```python
from build123d import *

# Parameters (mm, degrees)
F0_W      = 152.4
F0_H      = 91.581002
F1_DEPTH  = 50.8
F2_R      = 19.05
F3_DEPTH  = 152.4
F2_R_2    = 22.225
F4_DEPTH  = 6.35
F5_R      = 22.225
F5_R_2    = 19.05
F6_DEPTH  = 6.35
F7_R      = 19.05
F8_DEPTH  = 82.55
F10_R     = 6.35
F11_DEPTH = 152.4
F12_R     = 6.35
F13_DEPTH = 38.1


with BuildPart() as f1:
    # F0 (on Right) → F1 (new body, symmetric)
    with BuildSketch(Plane.YZ):
        Rectangle(F0_W, F0_H)
    extrude(amount=F1_DEPTH, both=True)

    # F2 (on face) → F3 (cut, symmetric)
    with BuildSketch(Plane(origin=(0, 76.2, 0), x_dir=(-1, 0, 0), z_dir=(0, 1, 0))):
        Circle(F2_R)
    extrude(amount=F3_DEPTH, both=True, mode=Mode.SUBTRACT)

    # F2 (on face) → F4 (cut)
    with BuildSketch(Plane(origin=(0, 76.2, 0), x_dir=(-1, 0, 0), z_dir=(0, 1, 0))):
        Circle(F2_R_2)
        Circle(F2_R, mode=Mode.SUBTRACT)
    extrude(amount=-F4_DEPTH, mode=Mode.SUBTRACT)

    # F5 (on face) → F6 (cut)
    with BuildSketch(Plane.XZ.offset(76.2)):
        Circle(F5_R)
        Circle(F5_R_2, mode=Mode.SUBTRACT)
    extrude(amount=-F6_DEPTH, mode=Mode.SUBTRACT)

    # F7 (on Front) → F8 (join, symmetric)
    with BuildSketch(Plane.XZ):
        Circle(F7_R)
    extrude(amount=F8_DEPTH, both=True)

    # F10 (on face) → F11 (cut)
    with BuildSketch(Plane(origin=(-50.8, 0, 0), x_dir=(0, -1, 0), z_dir=(-1, 0, 0))):
        Circle(F10_R)
    extrude(amount=-F11_DEPTH, mode=Mode.SUBTRACT)

    # F12 (on Right) → F13 (join, symmetric)
    with BuildSketch(Plane.YZ):
        Circle(F12_R)
    extrude(amount=F13_DEPTH, both=True)


solid = f1.part
```
For this review, take the finished solid that the model builds, in its own axes (mm). A direction names the side the tool comes from. Round coordinates to 2 decimals unless told otherwise and drop trailing zeros. Write each loop counter-clockwise with the first axis right and the second up, starting at its lowest first coordinate (ties: lowest second). Pieces come first, ordered by that corner, then holes. Notation, with made-up numbers: (78.5, 21) - (120.5, 21) arc R8 cw to (120.5, 28) - close; hole circle Ø3 at (5.25, -27.5). An arc over 180 degrees is marked (long way). Answer as CSV lines item,"result". Start each with the question number.
(1) Machinability: for faces 4 (the flat face through (0, -82.55, 0)), 5 (the flat face through (-16.4, 69.85, 10)), 6 (the flat face through (38.1, 0, 0)), 7 (the cylindrical face through (-44.54, 1.38, -6.2)), 8 (the cylindrical face through (21.199, -73.069, 6.676)), which of the approach directions +Z, -Z, +X, -X, +Y, -Y give a long, thin tool a straight path to every point of the face, cutting with its end or side? Answer none if there is none.
(2) For line 1 (Y direction, x = 47, z = 0); line 2 (Z direction, x = -44, y = 0); line 3 (Z direction, x = 13.5, y = 71.5), list the stretches that pass through material, from the lowest coordinate up.
(3) For pin 1 (1.5 mm diameter, centred on x = -26.5, z = -19.5, fed in from -Y); pin 2 (10 mm diameter, centred on x = -37, z = -5, fed in from +Y); pin 3 (11.5 mm diameter, centred on y = 0, z = 0, fed in from -X); pin 4 (14 mm diameter, centred on y = -0.5, z = 2.5, fed in from +X), all flat-tipped, find the tip position at first contact; note any pin that passes through.
(4) Mouldability with a two-part tool opening along Z and no side actions: class faces 1 (the flat face through (23, 76.2, -1)), 2 (the flat face through (1, -1, 45.791)), 3 (the cylindrical face through (-21.199, 73.069, 6.676)) as +Z half, -Z half, draft (parallel to the pull), parting line (faces both ways), or undercut.
(5) Add section A-A, the plane y = 0. State the section outline as (x, z) points, plus the area to 3 significant figures.
(6) Add section D-D, the plane z = 32.5. State the section outline as (x, y) points.
(7) Add section C-C, the plane z = 10. State the section outline as (x, y) points.
From the geometry:
1,face 4,"+Z, -Z, +X, -X, -Y"
1,face 5,"+Y"
1,face 6,"+X"
1,face 7,"-X"
1,face 8,"-Y"
2,line 1,"y = -76.2 to -6.35, 6.35 to 76.2"
2,line 2,"z = -45.79 to -6.35, 6.35 to 45.79"
2,line 3,"z = -45.79 to -17.66, -13.44 to 13.44, 17.66 to 45.79"
3,pin 1,"stops at y = -76.2"
3,pin 2,"stops at y = 76.2"
3,pin 3,"stops at x = -38.1"
3,pin 4,"stops at x = 50.8"
4,face 1,"draft"
4,face 2,"+Z half"
4,face 3,"undercut"
5,outline,"(-50.8, -45.79) - (50.8, -45.79) - (50.8, -6.35) - (38.1, -6.35) - (38.1, 6.35) - (50.8, 6.35) - (50.8, 45.79) - (-50.8, 45.79) - (-50.8, 6.35) - (-38.1, 6.35) - (-38.1, -6.35) - (-50.8, -6.35) - close"
5,area,"8,980 mm²"
6,outline,"(-50.8, -76.2) - (50.8, -76.2) - (50.8, 76.2) - (-50.8, 76.2) - close"
7,outline,"(-50.8, -76.2) - (-19.85, -76.2) - (-19.85, -69.85) - (-16.21, -69.85) - (-16.21, -82.55) - (16.21, -82.55) - (16.21, -69.85) - (19.85, -69.85) - (19.85, -76.2) - (50.8, -76.2) - (50.8, 76.2) - (19.85, 76.2) - (19.85, 69.85) - (16.21, 69.85) - (16.21, 82.55) - (-16.21, 82.55) - (-16.21, 69.85) - (-19.85, 69.85) - (-19.85, 76.2) - (-50.8, 76.2) - close"
